Design review of the part built by this model. Coordinates are the model's own, in mm. Give positions to 0.01 mm unless a question says otherwise; leave off trailing zeros. Loops run counter-clockwise (first coordinate to the right, second up) from the corner with the lowest first, then second, coordinate; pieces in that order, holes last. Notation, with made-up numbers: (42, 63.25) -> (54, 63.25) arc R14 cw to (54, 86.25) -> close; hole circle Ø8 at (79, -36.5). An arc over 180 degrees is marked (long way). Use a Markdown table: item, result. Add a question column.
1. Add section A-A (x = -127). State the section outline as (y, z) points.
2. Add section B-B (x = 136). State the section outline as (y, z) points.
3. Add section C-C (y = 2.05). Count the separate pieces of the cut face and the enclosed holes in it, and give its area (3 significant figures).
4. Add section D-D (z = -117.5). State the section outline as (x, y) points.
5. For pin 1 Ø1.5 at (y, z) = (2, -56.5) entering from -X; pin 2 Ø1.5 at (y, z) = (3, -156) entering from +X; pin 3 Ø2 at (x, z) = (-10, 72) entering from -Y; pin 4 Ø1.5 at (x, y) = (-18, 2.5) entering from -Z, all flat-tipped, find the tip position at first contact; note any pin that passes through.
6. To check wall thickness, follow line 1 (X direction, y = 1.4, z = 134); line 2 (X direction, y = 3.95, z = -39.25); line 3 (X direction, y = 3.25, z = 101.6). State the ranges of each line that lie inside material, in increasing order.
Autodesk Inventor part; units mm, degrees
ref_plane "YZ Plane" through (0, 0, 0) normal (1, 0, 0) x (0, 1, 0)
ref_plane "XZ Plane" through (0, 0, 0) normal (0, 1, 0) x (-1, 0, 0)
ref_plane "XY Plane" through (0, 0, 0) normal (0, 0, 1) x (1, 0, 0)
sketch "Sketch1" plane through (0, 0, 0) normal (0, 1, 0) x (-1, 0, 0)
  arc A0 (-177, 0) -> (177, 0) centre (0, 0) ccw
  line L0 (-177, 0) -> (-177, 151.6)
  line L1 (-151.6, 177) -> (151.6, 177)
  line L2 (177, 151.6) -> (177, 0)
  arc A1 (-151.6, 177) -> (-177, 151.6) centre (-151.6, 151.6) ccw
  arc A2 (177, 151.6) -> (151.6, 177) centre (151.6, 151.6) ccw
  point P0 (-177, 177)
  point P1 (177, 177)
  dimension "d0" = 354
  dimension "d98" = 177
  dimension "d99" = 177
  dimension "d101" = 354
  dimension "d102" = 177
  dimension "d217" = 25.4
extrude "Extrusion1" add sketch "Sketch1" along normal blind 5
sketch "Sketch8" plane through (0, 5, 0) normal (0, 1, 0) x (1, 0, 0)
  circle A0 centre (101.6, -101.6) radius 1.7
  circle A1 centre (101.6, 101.6) radius 1.7
  circle A2 centre (-101.6, 101.6) radius 1.7
  circle A3 centre (-101.6, -101.6) radius 1.7
  arc A4 (177, 0) -> (-177, 0) centre (0, 0) ccw construction
  line L0 (0, 177) -> (0, -177) construction
  line L1 (-151.6, -177) -> (151.6, -177) construction
  line L2 (-177, 0) -> (-177, -151.6) construction
  line L3 (177, -151.6) -> (177, 0) construction
  line L4 (-177, 0) -> (177, 0) construction
  circle A5 centre (0, -101.6) radius 1.7
  point P0 (0, 0)
  point P1 (-177, -177)
  point P2 (177, -177)
  dimension "d103" = 3.4
  dimension "d104" = 3.4
  dimension "d105" = 3.4
  dimension "d106" = 3.4
  dimension "d115" = 101.6
  dimension "d116" = 101.6
  dimension "d117" = 101.6
  dimension "d118" = 101.6
  dimension "d119" = 101.6
  dimension "d120" = 101.6
  dimension "d121" = 101.6
  dimension "d122" = 101.6
  dimension "d255" = 3.4
  dimension "d256" = 101.6
extrude "Stand-Offs" cut sketch "Sketch8" against normal through all
sketch "Sketch9" plane through (0, 5, 0) normal (0, 1, 0) x (1, 0, 0)
  line L0 (-150.65, -84.3) -> (-150.65, -164.3)
  line L1 (-150.65, -164.3) -> (-120.65, -164.3)
  line L2 (-120.65, -164.3) -> (-120.65, -84.3)
  line L3 (-120.65, -84.3) -> (-150.65, -84.3)
  circle A0 centre (-114.3, -98.9) radius 1.7
  circle A1 centre (-114.3, -149.7) radius 1.7
  circle A2 centre (-157, -149.7) radius 1.7
  circle A3 centre (-157, -98.9) radius 1.7
  arc A4 (177, 0) -> (-177, 0) centre (0, 0) ccw construction
  line L4 (0, 177) -> (0, -177) construction
  line L5 (-151.6, -177) -> (151.6, -177) construction
  line L6 (-120.65, -124.3) -> (-150.65, -124.3) construction
  line L7 (150.65, -164.3) -> (120.65, -164.3)
  line L8 (120.65, -164.3) -> (120.65, -84.3)
  line L9 (120.65, -84.3) -> (150.65, -84.3)
  circle A5 centre (114.3, -98.9) radius 1.7
  circle A6 centre (114.3, -149.7) radius 1.7
  line L10 (150.65, -84.3) -> (150.65, -164.3)
  circle A7 centre (157, -98.9) radius 1.7
  circle A8 centre (157, -149.7) radius 1.7
  line L11 (120.65, -124.3) -> (150.65, -124.3) construction
  line L12 (0, -177) -> (-236.8089, -177) construction
  point P0 (177, -177)
  point P1 (177.1241, 0)
  dimension "d126" = 30
  dimension "d129" = 3.4
  dimension "d130" = 3.4
  dimension "d131" = 3.4
  dimension "d132" = 3.4
  dimension "d133" = 6.35
  dimension "d134" = 6.35
  dimension "d135" = 6.35
  dimension "d136" = 6.35
  dimension "d141" = 120.65
  dimension "d143" = 80
  dimension "d144" = 25.4
  dimension "d145" = 25.4
  dimension "d146" = 25.4
  dimension "d147" = 25.4
  dimension "d236" = 12.7
extrude "Wheels" cut sketch "Sketch9" against normal through all
sketch "Sketch10" plane through (0, 5, 0) normal (0, 1, 0) x (1, 0, 0)
  circle A0 centre (-70.11, -137.7493) radius 1.7
  circle A1 centre (-28.3016, -137.7493) radius 1.7
  circle A2 centre (-70.11, -110.8507) radius 1.7
  circle A3 centre (-28.3016, -110.8507) radius 1.7
  arc A4 (177, 0) -> (-177, 0) centre (0, 0) ccw construction
  line L0 (0, 177) -> (0, -177) construction
  line L1 (-151.6, -177) -> (151.6, -177) construction
  line L2 (177, -151.6) -> (177, 0) construction
  line L3 (-177, 0) -> (-177, -151.6) construction
  line L4 (177, 0) -> (-177, 0) construction
  line L5 (-150.65, -84.3) -> (-150.65, -164.3) construction
  line L6 (-150.65, -124.3) -> (150.65, -124.3) construction
  line L7 (150.65, -84.3) -> (150.65, -164.3) construction
  line L8 (-120.65, -84.3) -> (-120.65, -164.3) construction
  circle A5 centre (70.11, -137.7493) radius 1.7
  circle A6 centre (70.11, -110.8507) radius 1.7
  circle A7 centre (28.3016, -137.7493) radius 1.7
  circle A8 centre (28.3016, -110.8507) radius 1.7
  point P0 (-177, -177)
  point P1 (177, -177)
  dimension "d150" = 3.4
  dimension "d151" = 3.4
  dimension "d152" = 3.4
  dimension "d153" = 3.4
  dimension "d154" = 26.8986
  dimension "d155" = 26.8986
  dimension "d156" = 41.8084
  dimension "d157" = 41.8084
  dimension "d161" = 50.54
  dimension "d162" = 13.4493
  dimension "d163" = 13.4493
  dimension "d166" = 13.4493
  dimension "d167" = 13.4493
extrude "Motor Mount" cut sketch "Sketch10" against normal through all
sketch "Sketch11" plane through (0, 5, 0) normal (0, 1, 0) x (1, 0, 0)
  circle A0 centre (-46.25, 39.25) radius 1.7
  circle A1 centre (46.25, 39.25) radius 1.7
  circle A2 centre (46.25, -39.25) radius 1.7
  circle A3 centre (-46.25, -39.25) radius 1.7
  line L0 (-177, 0) -> (-177, -151.6) construction
  arc A4 (177, 0) -> (-177, 0) centre (0, 0) ccw construction
  line L1 (-177, 0) -> (177, 0) construction
  line L2 (0, 177) -> (0, -177) construction
  line L3 (-151.6, -177) -> (151.6, -177) construction
  point P0 (-177, -177)
  point P1 (177, -177)
  dimension "d170" = 3.4
  dimension "d171" = 3.4
  dimension "d172" = 3.4
  dimension "d173" = 3.4
  dimension "d174" = 92.5
  dimension "d175" = 92.5
  dimension "d176" = 78.5
  dimension "d177" = 78.5
  dimension "d183" = 46.25
  dimension "d184" = 39.25
  dimension "d185" = 39.25
  dimension "d186" = 46.25
  dimension "d235" = 46.25
extrude "PCB" cut sketch "Sketch11" against normal through all
sketch "Sketch12" plane through (0, 5, 0) normal (0, 1, 0) x (1, 0, 0)
  circle A0 centre (95.25, 136.36) radius 1.7
  circle A1 centre (78.74, 99.9262) radius 1.7
  line L0 (-177, 0) -> (-177, -151.6) construction
  line L1 (-177, 0) -> (177, 0) construction
  arc A2 (177, 0) -> (-177, 0) centre (0, 0) ccw construction
  line L2 (78.74, 99.9262) -> (95.25, 136.36) construction
  circle A3 centre (-78.74, 99.9262) radius 1.7
  circle A4 centre (-95.25, 136.36) radius 1.7
  line L3 (0, 177) -> (0, 0) construction
  line L4 (115.2165, 177) -> (-115.2165, 177) construction
  circle A5 centre (101.6, 101.6) radius 1.7 construction
  circle A6 centre (-101.6, 101.6) radius 1.7 construction
  point P0 (-177, -177)
  dimension "d190" = 3.4
  dimension "d191" = 3.4
  dimension "d240" = 40
  dimension "d243" = 95.25
  dimension "d244" = 40
  dimension "d245" = 3.4
  dimension "d246" = 3.4
  dimension "d247" = 40.64
  dimension "d248" = 6.35
  dimension "d249" = 95.25
  dimension "d250" = 6.35
  dimension "d251" = 22.86
  dimension "d252" = 22.86
  dimension "d253" = 40.64
  dimension "d254" = 34.76
extrude "Ball Caster" cut sketch "Sketch12" against normal through all
sketch "Sketch13" plane through (0, 5, 0) normal (0, 1, 0) x (1, 0, 0)
  line L0 (-34.925, 157.4) -> (-28.575, 157.4)
  line L1 (-28.575, 157.4) -> (-28.575, 152.4)
  line L2 (-28.575, 152.4) -> (-34.925, 152.4)
  line L3 (-34.925, 152.4) -> (-34.925, 157.4)
  line L4 (-22.225, 157.4) -> (-15.875, 157.4)
  line L5 (-15.875, 157.4) -> (-15.875, 152.4)
  line L6 (-15.875, 152.4) -> (-22.225, 152.4)
  line L7 (-22.225, 152.4) -> (-22.225, 157.4)
  line L8 (-9.525, 157.4) -> (-3.175, 157.4)
  line L9 (-3.175, 157.4) -> (-3.175, 152.4)
  line L10 (-3.175, 152.4) -> (-9.525, 152.4)
  line L11 (-9.525, 152.4) -> (-9.525, 157.4)
  line L12 (3.175, 157.4) -> (9.525, 157.4)
  line L13 (9.525, 157.4) -> (9.525, 152.4)
  line L14 (9.525, 152.4) -> (3.175, 152.4)
  line L15 (3.175, 152.4) -> (3.175, 157.4)
  line L16 (15.875, 157.4) -> (22.225, 157.4)
  line L17 (22.225, 157.4) -> (22.225, 152.4)
  line L18 (22.225, 152.4) -> (15.875, 152.4)
  line L19 (15.875, 152.4) -> (15.875, 157.4)
  line L20 (28.575, 157.4) -> (34.925, 157.4)
  line L21 (34.925, 157.4) -> (34.925, 152.4)
  line L22 (34.925, 152.4) -> (28.575, 152.4)
  line L23 (28.575, 152.4) -> (28.575, 157.4)
  arc A0 (177, 0) -> (-177, 0) centre (0, 0) ccw construction
  line L24 (0, 177) -> (0, -177) construction
  line L25 (-151.6, -177) -> (151.6, -177) construction
  line L26 (177, -151.6) -> (177, 0) construction
  line L27 (-177, 0) -> (-177, -151.6) construction
  line L28 (177, 0) -> (-177, 0) construction
  point P0 (-177, -177)
  point P1 (177, -177)
  dimension "d204" = 5
  dimension "d205" = 6.35
  dimension "d208" = 12.7
  dimension "d213" = 152.4
  dimension "d214" = 3.175
extrude "Switch" cut sketch "Sketch13" against normal through all
equation "\"d101\" = d0"
equation "\"m3_heat_set_insert\" = 4"
equation "\"m3_clearance\" = 3.4"
equation "\"m3_heat_set_depth\" = 7"
equation "\"hardboard_thickness\" = 5"
equation "\"robot_diameter\" = 354"
equation "\"motor_centerline_height\" = 13"
properties part number "layer1"
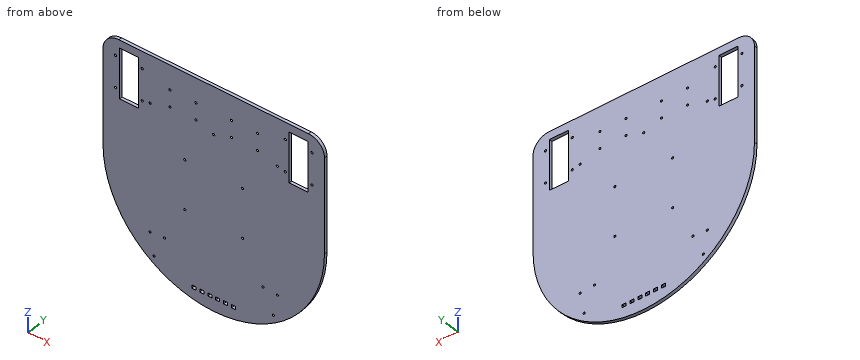
Taken from the geometry:
| question | item | result |
|---|---|---|
| 1 | outline | (0, -123.29) -> (5, -123.29) -> (5, 84.3) -> (0, 84.3) -> close; (0, 164.3) -> (5, 164.3) -> (5, 177) -> (0, 177) -> close |
| 2 | outline | (0, -113.28) -> (5, -113.28) -> (5, 84.3) -> (0, 84.3) -> close; (0, 164.3) -> (5, 164.3) -> (5, 177) -> (0, 177) -> close |
| 3 | separate pieces | 1 |
| 3 | enclosed holes | 37 |
| 3 | area | 106,000 mm^2 |
| 4 | outline | (-132.37, 0) -> (132.37, 0) -> (132.37, 5) -> (-132.37, 5) -> close |
| 5 | pin 1 | stops at x = -167.99 |
| 5 | pin 2 | stops at x = 85.01 |
| 5 | pin 3 | stops at y = 0 |
| 5 | pin 4 | stops at z = -176.16 |
| 6 | line 1 | x = -177 to -150.65, -120.65 to 120.65, 150.65 to 177 |
| 6 | line 2 | x = -172.59 to -47.95, -44.55 to 44.55, 47.95 to 172.59 |
| 6 | line 3 | x = -177 to -150.65, -120.65 to -103.3, -99.9 to -1.7, 1.7 to 99.9, 103.3 to 120.65, 150.65 to 177 |
